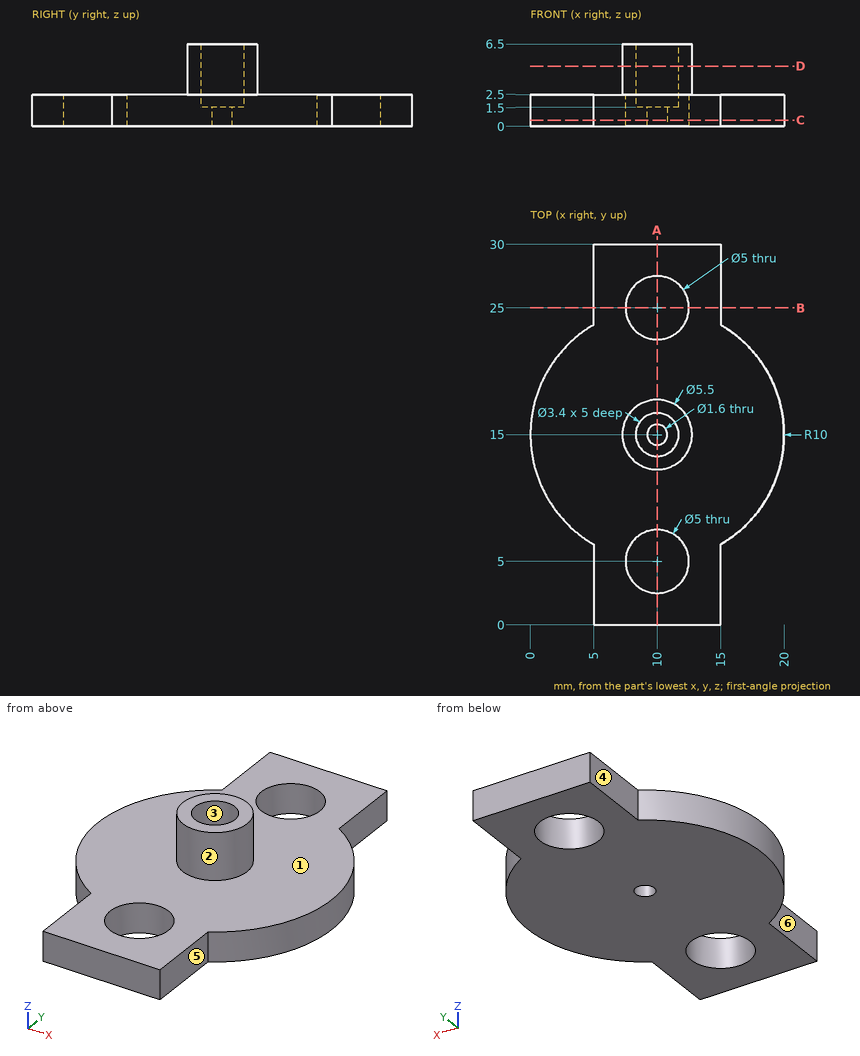
For this review, use the dimensioned drawing (mm, ordinates from the lowest corner) and the shaded views. A direction names the side the tool comes from. Give positions to 0.01 mm unless a question says otherwise; leave off trailing zeros. Order: outer loops, then holes, each group sorted by start corner. A loop starts at its lowest first (then second) coordinate and runs counter-clockwise, first axis right, second up. Notation, with made-up numbers: (-26, 13) -> (-14, 13) arc R11 ccw to (-14, 28) -> close; hole circle Ø10 at (25, -16.5). An arc over 180 degrees is marked (long way). Write item = value, one per line. Start each with the question number.
(1) Take a section at D-D (z = 4.75). Write out the cut boundary in (x, y).
(2) Tool access review of the marked faces 4, 5 and 6: name each direction out of +Z, -Z, +X, -X, +Y, -Y from which nothing blocks a thin tool from reaching the whole face with its end or side.
(3) Take a section at B-B (y = 25). Write out the cut boundary in (x, z), plus the area to 3 significant figures.
(4) For L1, parallel to Y at x = 10, z = 0.65; L2, parallel to Y at x = 10, z = 1.8; L3, parallel to Y at x = 10, z = 2.75, list the stretches that pass through material, from the lowest coordinate up. Write a range as from..to.
(5) For pin 1 Ø3 at (y, z) = (2.5, 1) entering from +X; pin 2 Ø2 at (y, z) = (23.5, 3) entering from +X; pin 3 Ø2 at (y, z) = (18.5, 1.5) entering from -X; pin 4 Ø6 at (x, y) = (10, 25) entering from -Z, all flat-tipped, find the tip position at first contact; note any pin that passes through.
(6) Take a section at C-C (z = 0.5). Write out the cut boundary in (x, y), plus the area to 3 significant figures.
(7) Take a section at A-A (x = 10). Write out the cut boundary in (y, z).
(8) Draft analysis for pull direction Y (two halves, no side actions). For the marked faces 1, 2 and 3, state which applies: +Y half, -Y half, draft (parallel to the pull), parting line (faces both ways), or undercut.
Returned:
q1.outline = circle Ø5.5 at (10, 15); hole circle Ø3.4 at (10, 15)
q2.face_4 = +Z, -Z, -X, +Y
q2.face_5 = +Z, -Z, +X, -Y
q2.face_6 = +Z, -Z, -X, -Y
q3.outline = (5, 0) -> (7.5, 0) -> (7.5, 2.5) -> (5, 2.5) -> close; (12.5, 0) -> (15, 0) -> (15, 2.5) -> (12.5, 2.5) -> close
q3.area = 12.5 mm²
q4.L1 = 0..2.5, 7.5..14.2, 15.8..22.5, 27.5..30
q4.L2 = 0..2.5, 7.5..13.3, 16.7..22.5, 27.5..30
q4.L3 = 12.25..13.3, 16.7..17.75
q5.pin_1 = 15
q5.pin_2 = 16.46
q5.pin_3 = 0.32
q5.pin_4 = 0
q6.outline = (5, 0) -> (15, 0) -> (15, 6.34) arc R10 ccw to (15, 23.66) -> (15, 30) -> (5, 30) -> (5, 23.66) arc R10 ccw to (5, 6.34) -> close; hole circle Ø5 at (10, 5); hole circle Ø5 at (10, 25); hole circle Ø1.6 at (10, 15)
q6.area = 382 mm²
q7.outline = (0, 0) -> (2.5, 0) -> (2.5, 2.5) -> (0, 2.5) -> close; (7.5, 0) -> (14.2, 0) -> (14.2, 1.5) -> (13.3, 1.5) -> (13.3, 6.5) -> (12.25, 6.5) -> (12.25, 2.5) -> (7.5, 2.5) -> close; (15.8, 0) -> (22.5, 0) -> (22.5, 2.5) -> (17.75, 2.5) -> (17.75, 6.5) -> (16.7, 6.5) -> (16.7, 1.5) -> (15.8, 1.5) -> close; (27.5, 0) -> (30, 0) -> (30, 2.5) -> (27.5, 2.5) -> close
q8.face_1 = draft
q8.face_2 = parting line
q8.face_3 = undercut
